```python
from build123d import *

# Parameters (mm, degrees)
SKETCH_R        = 12.5
PAD_DEPTH       = 24
SKETCH001_R     = 12.2
PAD001_DEPTH    = 30
SKETCH002_R     = 3.5
PAD002_DEPTH    = 2.5
SKETCH003_R     = 2
PAD003_DEPTH    = 9.5
SKETCH004_R     = 9
PAD004_DEPTH    = 7
SKETCH009_R     = 1.5
POCKET002_DEPTH = 3


with BuildPart() as part:
    # Sketch → Pad (new body)
    with BuildSketch(Plane.YZ):
        with Locations((20, 20)):
            Circle(SKETCH_R)
    extrude(amount=PAD_DEPTH)

    # Sketch001 (on Face3 of Pad) → Pad001 (join)
    with BuildSketch(Plane.YZ.offset(24)):
        with Locations((20, 20)):
            Circle(SKETCH001_R)
    extrude(amount=PAD001_DEPTH)

    # Sketch002 (on Face2 of Pad001) → Pad002 (join)
    with BuildSketch(Plane(origin=(0, 0, 0), x_dir=(0, 1, 0), z_dir=(-1, 0, 0))):
        with Locations((20, -20)):
            Circle(SKETCH002_R)
    extrude(amount=PAD002_DEPTH)

    # Sketch003 (on Face6 of Pad002) → Pad003 (join)
    with BuildSketch(Plane(origin=(-2.5, 0, 0), x_dir=(0, 1, 0), z_dir=(-1, 0, 0))):
        with Locations((20, -20)):
            Circle(SKETCH003_R)
    extrude(amount=PAD003_DEPTH)

    # Sketch004 (on Face7 of Pad003) → Pad004 (join)
    with BuildSketch(Plane.YZ.offset(54)):
        with Locations((20, 20)):
            Circle(SKETCH004_R)
    extrude(amount=PAD004_DEPTH)

    # Sketch009 (on Face2 of Pad004) → Pocket002 (cut)
    with BuildSketch(Plane(origin=(0, 0, 0), x_dir=(0, 1, 0), z_dir=(-1, 0, 0))):
        with Locations((28.5, -20)):
            Circle(SKETCH009_R)
        with Locations((11.5, -20)):
            Circle(SKETCH009_R)
    extrude(amount=-POCKET002_DEPTH, mode=Mode.SUBTRACT)


solid = part.part
```
The model under review builds one solid part; all positions refer to its coordinate system, in mm. A direction names the side the tool comes from. Round coordinates to 2 decimals unless told otherwise and drop trailing zeros. Loops run counter-clockwise (first coordinate to the right, second up) from the corner with the lowest first, then second, coordinate; pieces in that order, holes last.
1) Wall thickness on line 1 along X through (y, z) = (24, 30); line 2 along X through (y, z) = (12.5, 20.5); line 3 along Z through (x, y) = (0.7, 28.5): over which ranges is each line inside the solid? List them lowest first.
Values follow:
line 1: x = 0 to 54
line 2: x = 3 to 61
line 3: z = 10.83 to 18.5, 21.5 to 29.17
2) Consider section B-B on y = 20. State the section outline as (x, z) points.
Values follow:
outline: (-12, 18) - (-2.5, 18) - (-2.5, 16.5) - (0, 16.5) - (0, 7.5) - (24, 7.5) - (24, 7.8) - (54, 7.8) - (54, 11) - (61, 11) - (61, 29) - (54, 29) - (54, 32.2) - (24, 32.2) - (24, 32.5) - (0, 32.5) - (0, 23.5) - (-2.5, 23.5) - (-2.5, 22) - (-12, 22) - close
3) Consider section D-D on z = 12. State the section outline as (x, y) points, then the cut area to 3 significant figures.
Values follow:
outline: (0, 10.4) - (24, 10.4) - (24, 10.79) - (54, 10.79) - (54, 15.88) - (61, 15.88) - (61, 24.12) - (54, 24.12) - (54, 29.21) - (24, 29.21) - (24, 29.6) - (0, 29.6) - close
area: 1,070 mm2
4) Clearance check with flat-ended pins moving along their axes: P1, Ø6, axis at x = 34, y = 22.5, coming from the -Z side; P2, Ø3, axis at x = 3, y = 17.5, coming from the +Z side; P3, Ø5, axis at x = 28.5, z = 28.5, coming from the -Y side. State where each tip first meets the part, or that it passes through.
Values follow:
P1: stops at z = 7.8
P2: stops at z = 32.46
P3: stops at y = 9.38
5) Tool access review of faces 1 (the face through (-12, 20, 20)), 2 (the face through (3, 28, 20)), 3 (the face through (38.79, 25.63, 9.177)): name each direction out of +Z, -Z, +X, -X, +Y, -Y from which nothing blocks a thin tool from reaching the whole face with its end or side.
Values follow:
face 1: +Z, -Z, -X, +Y, -Y
face 2: -X
face 3: +X
6) The part is to be moulded in two halves that separate along Z. For faces 4 (the face through (-2.5, 22, 22)), 5 (the face through (-7, 20, 18)), 6 (the face through (3, 11, 20)), say which applies: pulls with the +Z half, pulls with the -Z half, needs draft (parallel to the pull), parting line crosses it, or undercut.
Values follow:
face 4: needs draft
face 5: parting line crosses it
face 6: undercut
7) Consider section C-C on x = 11. State the section outline as (y, z) points, then the cut area to 3 significant figures.
Values follow:
outline: circle Ø25 at (20, 20)
area: 491 mm2
8) Consider section A-A on z = 20. State the section outline as (x, y) points, then the cut area to 3 significant figures.
Values follow:
outline: (-12, 18) - (-2.5, 18) - (-2.5, 16.5) - (0, 16.5) - (0, 13) - (3, 13) - (3, 10) - (0, 10) - (0, 7.5) - (24, 7.5) - (24, 7.8) - (54, 7.8) - (54, 11) - (61, 11) - (61, 29) - (54, 29) - (54, 32.2) - (24, 32.2) - (24, 32.5) - (0, 32.5) - (0, 30) - (3, 30) - (3, 27) - (0, 27) - (0, 23.5) - (-2.5, 23.5) - (-2.5, 22) - (-12, 22) - close
area: 1,500 mm2
